from build123d import *

# Parameters (mm, degrees)
BOSS_EXTRUDE2_DEPTH            = 5
CHAMFER1_SIZE                  = 1
CBORE_FOR_M2_SHCS1_D           = 2.4
CBORE_FOR_M2_SHCS1_CBORE_D     = 4.4
CBORE_FOR_M2_SHCS1_CBORE_DEPTH = 2
FILLET2_R                      = 1.5
CBORE_FOR_M2_SHCS3_D           = 2.4
CBORE_FOR_M2_SHCS3_CBORE_D     = 4.4
CBORE_FOR_M2_SHCS3_CBORE_DEPTH = 2


with BuildPart() as part:
    # Sketch1 → Boss-Extrude2 (new body)
    with BuildSketch(Plane(origin=(0, 0, 0), x_dir=(1, 0, 0), z_dir=(0, 1, 0))):
        Polygon((0, 0), (0, 7.75), (7.75, 7.75), (7.75, 5.25), (2.5, 5.25), (2.5, 0), align=None)
    extrude(amount=BOSS_EXTRUDE2_DEPTH)

    # Chamfer1
    chamfer1_edges = [part.edges().sort_by_distance(p)[0] for p in [
        (0, 2.5, -7.75),
    ]]
    chamfer(chamfer1_edges, length=CHAMFER1_SIZE)

    # CBORE for M2 SHCS1 (through all)
    with Locations(Plane(origin=(0, 0, -7.75), x_dir=(-1, 0, 0), z_dir=(0, 0, -1))):
        with Locations((-5.25, 2.5)):
            CounterBoreHole(CBORE_FOR_M2_SHCS1_D / 2, CBORE_FOR_M2_SHCS1_CBORE_D / 2, CBORE_FOR_M2_SHCS1_CBORE_DEPTH)

    # Fillet2
    fillet2_edges = [part.edges().sort_by_distance(p)[0] for p in [
        (7.75, 5, -6.5),
        (1.25, 5, 0),
        (7.75, 0, -6.5),
        (1.25, 0, 0),
    ]]
    fillet(fillet2_edges, radius=FILLET2_R)

    # CBORE for M2 SHCS3 (through all)
    with Locations(Plane(origin=(2.5, 0, 0), x_dir=(0, 0, -1), z_dir=(1, 0, 0))):
        with Locations((2.5, 2.5)):
            CounterBoreHole(CBORE_FOR_M2_SHCS3_D / 2, CBORE_FOR_M2_SHCS3_CBORE_D / 2, CBORE_FOR_M2_SHCS3_CBORE_DEPTH)


solid = part.part
The listing builds one solid part. Answer for the finished solid, in the listing's coordinates (mm). A direction names the side the tool comes from. Give positions to 0.01 mm unless a question says otherwise; leave off trailing zeros. Order: outer loops, then holes, each group sorted by start corner. A loop starts at its lowest first (then second) coordinate and runs counter-clockwise, first axis right, second up. Notation, with made-up numbers: (82.25, 39) - (114.25, 39) arc R17 ccw to (114.25, 60) - close; hole circle Ø2 at (74, 46). An arc over 180 degrees is marked (long way). Answer as CSV lines item,"result".
Q1. Which of the six approach directions +Z, -Z, +X, -X, +Y, -Y give full straight-line access (tool end or side, diameter ignored) to faces 1 (the face through (1.23, 0.43, -0.45)), 2 (the face through (0.25, 3.51, -1.85)), 3 (the face through (1.51, 4.68, -2.21)), 4 (the face through (2.5, 2, -5)), 5 (the face through (3.8, 2.5, -5.75))?
Answer key:
face 1,"+Z, +X, -X, -Y"
face 2,"+X, -X"
face 3,"+X"
face 4,"+Z, +X, +Y, -Y"
face 5,"-Z"
Q2. A cutting plane is placed at B-B, the plane y = 2.35. Determine the outline of the cut face in (x, z).
Answer key:
outline,"(0, -6.75) - (1, -7.75) - (3.06, -7.75) - (3.06, -5.75) - (4.06, -5.75) - (4.06, -5.25) - (2.5, -5.25) - (2.5, -4.69) - (0.5, -4.69) - (0.5, -3.69) - (0, -3.69) - close; (0, -1.31) - (0.5, -1.31) - (0.5, -0.31) - (2.5, -0.31) - (2.5, 0) - (0, 0) - close; (6.44, -5.75) - (7.44, -5.75) - (7.44, -7.75) - (7.75, -7.75) - (7.75, -5.25) - (6.44, -5.25) - close"
Q3. Straight lines are drawn through the part: L1, parallel to Y at x = 0.25, z = -2.5; L2, parallel to Y at x = 5.25, z = -6.7; L3, parallel to X at y = 1.1, z = -5. For each, find the intervals that lie inside material, in ascending order.
Answer key:
L1,"y = 0 to 1.3, 3.7 to 5"
L2,"y = 0 to 0.3, 4.7 to 5"
L3,"x = 0 to 2.5"
Q4. A cutting plane is placed at A-A, the plane x = 1.75. Determine the outline of the cut face in (y, z).
Answer key:
outline,"(0, -7.75) - (5, -7.75) - (5, -1.5) arc R1.5 ccw to (3.5, 0) - (1.5, 0) arc R1.5 ccw to (0, -1.5) - close; hole circle Ø4.4 at (2.5, -2.5)"
Q5. A cutting plane is placed at C-C, the plane z = -2.5. Determine the outline of the cut face in (x, y).
Answer key:
outline,"(0, 0) - (2.5, 0) - (2.5, 0.3) - (0.5, 0.3) - (0.5, 1.3) - (0, 1.3) - close; (0, 3.7) - (0.5, 3.7) - (0.5, 4.7) - (2.5, 4.7) - (2.5, 5) - (0, 5) - close"
Q6. Each of these flat-tipped pins is pushed along its axis until it touches: pin 1 Ø3 at (x, y) = (5.25, 2.5) entering from +Z; pin 2 Ø3 at (y, z) = (0.5, -2.5) entering from +X; pin 3 Ø1.3 at (x, y) = (4.5, 2.5) entering from -Z. Where does it stop, or does it pass through?
Answer key:
pin 1,"stops at z = -5.25"
pin 2,"stops at x = 2.5"
pin 3,"stops at z = -5.75"
Q7. Determine the mould class of faces 6 (the face through (7.3, 0.43, -6.48)), 7 (the face through (1, 2, 0)), 8 (the face through (1.23, 4.55, -0.43)), 9 (the face through (3.15, 3.16, -6.76)) for opening direction Y: pulls with the +Y half, pulls with the -Y half, needs draft (parallel to the pull), parting line crosses it, or undercut.
Answer key:
face 6,"pulls with the -Y half"
face 7,"needs draft"
face 8,"pulls with the +Y half"
face 9,"undercut"
Q8. A cutting plane is placed at D-D, the plane x = 5.25. Determine the outline of the cut face in (y, z).
Answer key:
outline,"(0, -7.75) - (0.3, -7.75) - (0.3, -5.75) - (1.3, -5.75) - (1.3, -5.25) - (0, -5.25) - close; (3.7, -5.75) - (4.7, -5.75) - (4.7, -7.75) - (5, -7.75) - (5, -5.25) - (3.7, -5.25) - close"
